Autodesk Inventor part; units mm, degrees
ref_plane "Work Plane1" through (30.1625, 0, 0) normal (0, 0, -1) x (1, 0, 0)
ref_plane "YZ Plane" through (0, 0, 0) normal (1, 0, 0) x (0, 1, 0)
ref_plane "XZ Plane" through (0, 0, 0) normal (0, 1, 0) x (-1, 0, 0)
sketch "Skizze1" plane through (0, 0, 0) normal (0, 0, 1) x (1, 0, 0)
  line L0 (-0.9, 0) -> (8, 0)
  line L1 (8, 0) -> (8, 0.7)
  line L2 (8, 0.7) -> (0.6, 0.7)
  line L3 (0.6, 0.7) -> (0.4159, 0.6188)
  line L4 (0.4159, 0.6188) -> (0, 0.6188)
  line L5 (0, 0.6188) -> (0, 1.3)
  line L6 (-2.68, 0) -> (9.78, 0)
  line L7 (0, -0.26) -> (0, 1.56)
  line L8 (-0.9, 0) -> (-0.9, 1.2213)
  line L9 (0, 1.3) -> (-0.9, 1.2213)
  line L10 (0.6, 0.7) -> (0, 0.7) construction
  dimension "d0" = 8
  dimension "d1" = 7.4
  dimension "d2" = 0.1841
  dimension "d3" = 0.9
  dimension "d4" = 1.4
  dimension "d5" = 1.2376
  dimension "d9" = 2.6
  dimension "d10" = 5
revolve "Körper" add sketch "Skizze1" angle 360 about axis through (-0.9, 0, 0) along (1, 0, 0)
sketch "Skizze2" plane through (-0.9, 0, 0) normal (-1, 0, 0) x (0, 0, 1)
  circle A0 centre (0, 0) radius 1.3
  line L0 (0, 0) -> (0, 1.2213)
  line L1 (-1.3, 0.15) -> (1.3, 0.15)
  line L2 (1.3, 0.15) -> (1.3, -0.15)
  line L3 (1.3, -0.15) -> (-1.3, -0.15)
  line L4 (-1.3, -0.15) -> (-1.3, 0.15)
  line L5 (-1.3, 0) -> (1.3, 0) construction
  line L6 (0, 0.15) -> (0, -0.15) construction
  dimension "d11" = 0.3
  dimension "d12" = 2.6
fillet "Rundung1" radius 0.1 1 edges at (-0.9, -1.2213, 0)
extrude "Loch" cut sketch "Skizze2" against normal blind 0.4 contours A0 L3 L1 | L2 L3 A0 | A0 L1 L2 | A0 L4 L1 | L3 L4 A0
thread "Gewinde"
chamfer "Fase1" distance 0.1624 distance2 0.1841 1 edges at (8, -0.7, 0) measured on face at (8, 0.4293, -0.1327)
ref_plane "Work Plane1" through (30.1625, 0, 0) normal (0, 0, -1) x (1, 0, 0)
equation "\"d11\" = SBR"
equation "\"d12\" = KOD"
equation "\"d14\" = RR"
equation "\"d19\" = STI"
equation "\"d15\" = GEL"
equation "\"d17\" = -0.5 * SPD + 0.5 * GD"
equation "\"d0\" = NLG"
equation "\"d1\" = GEL"
equation "\"d3\" = KOH"
equation "\"d4\" = GD"
equation "\"d5\" = BDM"
equation "\"d9\" = KOD"
equation "\"d10\" = KEWI"
equation "\"GD\" = 1.4"
equation "\"NLG\" = 8"
equation "\"GEL\" = 7.4"
equation "\"KOD\" = 2.6"
equation "\"KOH\" = 0.9"
equation "\"GAL\" = 0.61345 * PTC"
equation "\"SPD\" = 1.07524"
equation "\"BDM\" = 1.23762"
equation "\"GUL\" = 0.61345 * PTC"
equation "\"RR\" = 0.1"
equation "\"SBR\" = 0.3"
equation "\"STI\" = 0.4"
equation "\"KEWI\" = 5deg"
equation "\"PTC\" = 0.3"
equation "\"THREADDIA\" = 1.4"
equation "\"TOA\" = 30deg"
equation "\"NND\" = 1.4"
equation "\"GD1\" = THREADDIA - 1.2269 * PTC"
properties part number "DIN 84 - M1,4 x 8" material "Stahl, weich"
Build history of the part. All positions in model axes, mm. A direction names the side the tool comes from. Give positions to 0.01 mm unless a question says otherwise; leave off trailing zeros. Order: outer loops, then holes, each group sorted by start corner. A loop starts at its lowest first (then second) coordinate and runs counter-clockwise, first axis right, second up. Notation, with made-up numbers: M -36.75,2.5 L -0.75,2.5 A30 ccw -0.75,28.5 Z; hole C 5,75 d9. An arc over 180 degrees is marked long. Use one line per item in the form item = value.
Q1. Which spindle directions (+Z, -Z, +X, -X, +Y, -Y) get a long thin tool onto all of the face, cutting with end or side? Do faces 1 (the cylindrical face through (4.2, -0.7, 0)), 2 (the conical face through (-0.489, -0.998, -0.765)), 3 (the cylindrical face through (0.21, 0.59, -0.19)). Say none if no direction does.
Conclusion:
face_1 = +X
face_2 = -X
face_3 = none
Q2. Slice it at B-B, the plane y = 0. Write the cut outline in (x, z).
Conclusion:
outline = M -0.5,-1.26 L 0,-1.3 L 0,-0.62 L 0.42,-0.62 L 0.6,-0.7 L 7.82,-0.7 L 8,-0.54 L 8,0.54 L 7.82,0.7 L 0.6,0.7 L 0.42,0.62 L 0,0.62 L 0,1.3 L -0.5,1.26 Z
Q3. Slice it at C-C, the plane x = 4.25. Write the cut outline in (y, z), and give its area (3 significant figures).
Conclusion:
outline = C 0,0 d1.4
area = 1.54 mm2
Q4. Wall check: probe 1 along X at (y, z) = (-0.9, -0.3); probe 2 along X at (y, z) = (0.1, -0.35); probe 3 along Z at (x, y) = (6.75, 0). Give the ranges that are in metal, low to high.
Conclusion:
probe_1 = -0.9 to 0
probe_2 = -0.5 to 8
probe_3 = -0.7 to 0.7
Q5. Pin check, flat tips, straight feed: P1, Ø1, axis at x = 6.5, y = 0, coming from the +Z side; P2, Ø1, axis at x = 2, z = 0, coming from the +Y side; P3, Ø1, axis at x = 7, y = 1, coming from the +Z side. Stop position of each tip, or through.
Conclusion:
P1 = 0.7
P2 = 0.7
P3 = 0.49
Q6. Slice it at A-A, the plane z = 0. Write the cut outline in (x, y), and give its area (3 significant figures).
Conclusion:
outline = M -0.9,-1.13 A0.1 ccw -0.81,-1.23 L 0,-1.3 L 0,-0.62 L 0.42,-0.62 L 0.6,-0.7 L 7.82,-0.7 L 8,-0.54 L 8,0.54 L 7.82,0.7 L 0.6,0.7 L 0.42,0.62 L 0,0.62 L 0,1.3 L -0.81,1.23 A0.1 ccw -0.9,1.13 L -0.9,0.15 L -0.5,0.15 L -0.5,-0.15 L -0.9,-0.15 Z
area = 13.2 mm2
